Input: part model. Units: mm. Frame: model coordinates. A direction names the side the tool comes from. Coordinates: 2 decimals unless noted, no trailing zeros. Order: outer loops, then holes, each group sorted by start corner. A loop starts at its lowest first (then second) coordinate and runs counter-clockwise, first axis right, second up. Notation, with made-up numbers: (46, 28.25) -> (81, 28.25) arc R17 cw to (81, 49.25) -> close; hole circle Ø2 at (76, 84.25). An arc over 180 degrees is marked (long way). One line per question, with ' | ' between items.
```python
from build123d import *

# Parameters (mm, degrees)
SALIENTE_EXTRUIR2_DEPTH = 12.7
SALIENTE_EXTRUIR4_DEPTH = 12.7
CROQUIS7_R              = 12.7
CORTAR_EXTRUIR1_DEPTH   = 12.7
SALIENTE_EXTRUIR5_DEPTH = 12.7
CROQUIS9_R              = 12.7
CORTAR_EXTRUIR2_DEPTH   = 28.702
CROQUIS10_R             = 12.7
CORTAR_EXTRUIR3_DEPTH   = 32.004


with BuildPart() as part:
    # Croquis1 → Saliente-Extruir2 (new body)
    with BuildSketch(Plane(origin=(0, 0, 0), x_dir=(1, 0, 0), z_dir=(0, 1, 0))):
        with BuildLine():
            Line((0, 0), (0, 50.8))
            Line((0, 50.8), (-88.9, 50.8))
            Line((-88.9, 50.8), (-88.9, 50.782381867))
            ThreePointArc((-88.9, 50.782381867), (-114.968896843, 25.391190933), (-88.9, 0))
            Line((-88.9, 0), (0, 0))
        make_face()
    extrude(amount=SALIENTE_EXTRUIR2_DEPTH)

    # Croquis5 → Saliente-Extruir4 (add)
    with BuildSketch(Plane.XY):
        with BuildLine():
            Line((0, 12.7), (0, 38.1))
            Line((0, 38.1), (-0.002616662, 38.1))
            ThreePointArc((-0.002616662, 38.1), (-19.05, 57.147383338), (-38.097383338, 38.1))
            Line((-38.097383338, 38.1), (-38.1, 38.1))
            Line((-38.1, 38.1), (-38.1, 12.7))
            Line((-38.1, 12.7), (0, 12.7))
        make_face()
    extrude(amount=-SALIENTE_EXTRUIR4_DEPTH)

    # Croquis7 → Cortar-Extruir1 (cut)
    with BuildSketch(Plane.XY):
        with Locations((-19.05, 38.1)):
            Circle(CROQUIS7_R)
    extrude(amount=-CORTAR_EXTRUIR1_DEPTH, mode=Mode.SUBTRACT)

    # Croquis8 → Saliente-Extruir5 (add)
    with BuildSketch(Plane(origin=(0, 0, -50.8), x_dir=(-1, 0, 0), z_dir=(0, 0, -1))):
        with BuildLine():
            Line((38.1, 12.7), (38.097383338, 38.1))
            ThreePointArc((38.097383338, 38.1), (19.048691669, 57.148691669), (0, 38.1))
            Line((0, 38.1), (0, 12.7))
            Line((0, 12.7), (38.1, 12.7))
        make_face()
    extrude(amount=-SALIENTE_EXTRUIR5_DEPTH)

    # Croquis9 → Cortar-Extruir2 (cut)
    with BuildSketch(Plane(origin=(0, 0, -50.8), x_dir=(-1, 0, 0), z_dir=(0, 0, -1))):
        with Locations((18.60399445, 37.760816035)):
            Circle(CROQUIS9_R)
    extrude(amount=-CORTAR_EXTRUIR2_DEPTH, mode=Mode.SUBTRACT)

    # Croquis10 → Cortar-Extruir3 (cut)
    with BuildSketch(Plane(origin=(0, 12.7, 0), x_dir=(1, 0, 0), z_dir=(0, 1, 0))):
        with Locations(Location((-89.568896843, 25.391190933, 0), (0, 0, 270))):
            Circle(CROQUIS10_R)
    extrude(amount=-CORTAR_EXTRUIR3_DEPTH, mode=Mode.SUBTRACT)


solid = part.part
```
1. Access query for faces 4 (the face through (-19, 25, -12.7)), 5 (the face through (-35, 16, 0)), 6 (the face through (-38.1, 26, -6)), 7 (the face through (-15.851, 25.363, -44.539)), 8 (the face through (-12.223, 48.809, -6.261)). Directions: +Z, -Z, +X, -X, +Y, -Y. A direction counts if a zero-diameter tool reaches every point of the face in a straight line with its end or side. Return the directions, or none.
Recorded:
face 4: +X, -X, +Y | face 5: +Z, +X, -X, +Y, -Y | face 6: +Z, -Z, -X, +Y | face 7: -Z | face 8: +Z
2. Cut plane B-B, the plane y = 30. Return loops of the section in (x, z), and give its area (3 significant figures).
Recorded:
outline: (-38.1, -50.8) -> (-28.66, -50.8) -> (-28.66, -38.1) -> (-38.1, -38.1) -> close; (-38.1, -12.7) -> (-28.83, -12.7) -> (-28.83, 0) -> (-38.1, 0) -> close; (-9.27, -12.7) -> (0, -12.7) -> (0, 0) -> (-9.27, 0) -> close; (-8.55, -50.8) -> (0, -50.8) -> (0, -38.1) -> (-8.55, -38.1) -> close | area: 464 mm^2
3. Cut plane A-A, the plane x = -19.05. Return loops of the section in (y, z), and give its area (3 significant figures).
Recorded:
outline: (0, -50.8) -> (25.07, -50.8) -> (25.07, -38.1) -> (12.7, -38.1) -> (12.7, -12.7) -> (25.4, -12.7) -> (25.4, 0) -> (0, 0) -> close; (50.45, -50.8) -> (57.15, -50.8) -> (57.15, -38.1) -> (50.45, -38.1) -> close; (50.8, -12.7) -> (57.15, -12.7) -> (57.15, 0) -> (50.8, 0) -> close | area: 1,130 mm^2
4. Pin query (flat end, axial travel): pin 1 Ø6 at (y, z) = (6.5, -41) entering from -X; pin 2 Ø6 at (x, y) = (-98, 13) entering from -Z; pin 3 Ø15 at (x, z) = (-67.5, -19) entering from +Y; pin 4 Ø1 at (y, z) = (51, -37.5) entering from -X. Return the tip coordinate at first contact, or that it passes through.
Recorded:
pin 1: stops at x = -111.62 | pin 2: stops at z = -50.2 | pin 3: stops at y = 12.7 | pin 4: passes through
5. Ray query, line 1 (Z direction, x = -8, y = 18); line 2 (X direction, y = 38, z = -12); line 3 (Y direction, x = -19.05, z = -7.25). Return the intervals inside material, ascending. Write a range as [from, to].
Recorded:
line 1: z = [-50.8, -38.1], [-12.7, 0] | line 2: x = [-38.1, -31.75], [-6.35, 0] | line 3: y = [0, 25.4], [50.8, 57.15]
6. Cut plane D-D, the plane x = -92. Return loops of the section in (y, z).
Recorded:
outline: (0, -50.67) -> (12.7, -50.67) -> (12.7, -37.86) -> (0, -37.86) -> close; (0, -12.93) -> (12.7, -12.93) -> (12.7, -0.11) -> (0, -0.11) -> close
7. Mould query, pull axis Z, two halves, no side actions, for faces 1 (the face through (-18.631, 57.143, -6.261)), 2 (the face through (-58, 12.7, -26)), 3 (the face through (-114.963, 6.261, -25.959)). Classes: released by +Z, released by -Z, zero draft, split by the parting line, or undercut.
Recorded:
face 1: zero draft | face 2: undercut | face 3: split by the parting line
